from build123d import *

# Parameters (mm, degrees)
F0_W     = 20
F0_H     = 20
F1_DEPTH = 110
F2_W     = 20
F2_H     = 10
F3_DEPTH = 20
F4_W     = 180
F4_H     = 10
F5_DEPTH = 20


with BuildPart() as f1:
    # F0 (on Right) → F1 (new body, symmetric)
    with BuildSketch(Plane.YZ):
        Rectangle(F0_W, F0_H)
    extrude(amount=F1_DEPTH, both=True)

    # F2 (on face) → F3 (cut)
    with BuildSketch(Plane.XZ.offset(10)):
        with Locations((0, 5)):
            Rectangle(F2_W, F2_H)
    extrude(amount=-F3_DEPTH, mode=Mode.SUBTRACT)

    # F4 (on face) → F5 (cut)
    with BuildSketch(Plane.XY.offset(10)):
        with Locations((0, 5)):
            Rectangle(F4_W, F4_H)
    extrude(amount=-F5_DEPTH, mode=Mode.SUBTRACT)


solid = f1.part
Read the model definition and answer for the solid it produces. Units are mm, in the model's axes. A direction names the side the tool comes from. Coordinates: 2 decimals unless noted, no trailing zeros. Loops run counter-clockwise (first coordinate to the right, second up) from the corner with the lowest first, then second, coordinate; pieces in that order, holes last. Notation, with made-up numbers: (51, 62) - (94, 62) arc R16 cw to (94, 76) - close; hole circle Ø11 at (77, -14.75). An arc over 180 degrees is marked (long way). Answer in a Markdown table with one row per item.
Q1. For faces 4 (the flat face through (-10, -5, 5)), 5 (the flat face through (-70, -2, 10)), 6 (the flat face through (-1, 0, -2)), determine the directions among +Z, -Z, +X, -X, +Y, -Y from which every point of the face is accessible in a straight line to the end or side of a thin tool.
Here are the results:
| item | result |
|---|---|
| face 4 | +Z, +Y, -Y |
| face 5 | +Z, +X, -X, +Y, -Y |
| face 6 | +Z, -Z, +Y |
Q2. Find section D-D on x = 13.5. Write down the section's boundary in (y, z), plus the area to 3 significant figures.
Here are the results:
| item | result |
|---|---|
| outline | (-10, -10) - (0, -10) - (0, 10) - (-10, 10) - close |
| area | 200 mm^2 |
Q3. Straight lines are drawn through the part: line 1 along X through (y, z) = (9.25, -7.25); line 2 along X through (y, z) = (-1, 1.5); line 3 along Y through (x, z) = (-80, 4). For each, find the intervals that lie inside material, in ascending order. Write a range as [from, to].
Here are the results:
| item | result |
|---|---|
| line 1 | x = [-110, -90], [90, 110] |
| line 2 | x = [-110, -10], [10, 110] |
| line 3 | y = [-10, 0] |
Q4. The mould has two halves that part along X. Classify faces 1 (the flat face through (-90, 5, 0)), 2 (the flat face through (72, -2, 10)), 3 (the flat face through (-110, 0, 0)): pulls with the +X half, pulls with the -X half, needs draft (parallel to the pull), parting line crosses it, or undercut.
Here are the results:
| item | result |
|---|---|
| face 1 | undercut |
| face 2 | needs draft |
| face 3 | pulls with the -X half |
Q5. Find section B-B on z = 3. Write down the section's boundary in (x, y).
Here are the results:
| item | result |
|---|---|
| outline | (-110, -10) - (-10, -10) - (-10, 0) - (-90, 0) - (-90, 10) - (-110, 10) - close; (10, -10) - (110, -10) - (110, 10) - (90, 10) - (90, 0) - (10, 0) - close |
Q6. Given P1, Ø1.5, axis at x = -86.5, z = 3, coming from the +Y side; P2, Ø10, axis at x = 86, z = -5.5, coming from the +Y side; P3, Ø11, axis at x = -3, y = -2.5, coming from the +Z side, each flat-ended and moving along its own axis, determine where each tip first touches the part or whether it passes through.
Here are the results:
| item | result |
|---|---|
| P1 | stops at y = 0 |
| P2 | stops at y = 10 |
| P3 | stops at z = 0 |
Q7. Find section C-C on y = -6. Write down the section's boundary in (x, z).
Here are the results:
| item | result |
|---|---|
| outline | (-110, -10) - (110, -10) - (110, 10) - (10, 10) - (10, 0) - (-10, 0) - (-10, 10) - (-110, 10) - close |
Q8. Find section A-A on y = 3.25. Write down the section's boundary in (x, z), plus the area to 3 significant figures.
Here are the results:
| item | result |
|---|---|
| outline | (-110, -10) - (-90, -10) - (-90, 10) - (-110, 10) - close; (90, -10) - (110, -10) - (110, 10) - (90, 10) - close |
| area | 800 mm^2 |
